Source: CAD feature listing. Evaluate the final solid. Frame: model axes, mm. A direction names the side the tool comes from. Round coordinates to 2 decimals unless told otherwise and drop trailing zeros. Loops run counter-clockwise (first coordinate to the right, second up) from the corner with the lowest first, then second, coordinate; pieces in that order, holes last. Notation, with made-up numbers: (77, 70.5) -> (125, 70.5) arc R9 cw to (125, 87.5) -> close; hole circle Ø8 at (45, 69). An arc over 180 degrees is marked (long way). Write item = value, one per line.
Autodesk Inventor part; units mm, degrees
ref_plane "YZ Plane" through (0, 0, 0) normal (1, 0, 0) x (0, 1, 0)
ref_plane "XZ Plane" through (0, 0, 0) normal (0, 1, 0) x (-1, 0, 0)
ref_plane "XY Plane" through (0, 0, 0) normal (0, 0, 1) x (1, 0, 0)
sketch "Sketch1" plane through (0, 0, 0) normal (0, 1, 0) x (-1, 0, 0)
  line L0 (0, 0) -> (31, 0)
  line L1 (31, 0) -> (31, -30)
  line L2 (31, -30) -> (28, -30)
  line L3 (28, -30) -> (28, -3)
  line L4 (28, -3) -> (0, -3)
  line L5 (0, -3) -> (0, 0) construction
  line L6 (0, 0) -> (-31, 0)
  line L7 (-31, 0) -> (-31, -30)
  line L8 (-31, -30) -> (-28, -30)
  line L9 (-28, -30) -> (-28, -3)
  line L10 (-28, -3) -> (0, -3)
  dimension "d0" = 31
  dimension "d1" = 30
  dimension "d2" = 3
  dimension "d3" = 27
extrude "Extrusion1" add sketch "Sketch1" along normal blind 20
sketch "Sketch2" plane through (31, 0, 0) normal (1, 0, 0) x (0, 0, -1)
  line L0 (30, 0) -> (0, 0) construction
  line L1 (0, 0) -> (15, 0) construction
  line L2 (15, 0) -> (15, 10) construction
  circle A0 centre (15, 10) radius 2.5
  dimension "d6" = 15
  dimension "d7" = 10
  dimension "d8" = 5
extrude "Extrusion2" cut sketch "Sketch2" against normal blind 70
fillet "Fillet1" radius 5 4 edges at (29.5, 20, -30) (29.5, 0, -30) (-29.5, 0, -30) (-29.5, 20, -30)
sketch "Sketch3" plane through (28, 0, -3) normal (0, 0, -1) x (-1, 0, 0)
  line L0 (28, 0) -> (28, 10) construction
  line L1 (28, 10) -> (48, 10) construction
  circle A0 centre (48, 10) radius 2
  circle A1 centre (8, 10) radius 2
  dimension "d12" = 10
  dimension "d13" = 20
  dimension "d14" = 4
extrude "Extrusion3" cut sketch "Sketch3" against normal blind 10
properties part number "Aligner"
1. Section query D-D (z = -15). Return the cut outline in (x, y).
Evaluation:
outline = (-31, 0) -> (-28, 0) -> (-28, 7.5) -> (-31, 7.5) -> close; (-31, 12.5) -> (-28, 12.5) -> (-28, 20) -> (-31, 20) -> close; (28, 0) -> (31, 0) -> (31, 7.5) -> (28, 7.5) -> close; (28, 12.5) -> (31, 12.5) -> (31, 20) -> (28, 20) -> close
2. Contact query for a flat-ended pin moving along its axis: pin 1 Ø4.5 at (x, y) = (-20, 10) entering from -Z. Output: stop coordinate, or through.
Evaluation:
pin_1 = -3
3. Line query: probe 1 along X at (y, z) = (9, -4.5); probe 2 along Y at (x, z) = (20, -1.7); probe 3 along Z at (x, y) = (10, 8). Output: solid intervals per line, ascending. Write a range as from..to.
Evaluation:
probe_1 = -31..-28, 28..31
probe_2 = 0..8, 12..20
probe_3 = -3..0
4. Section query A-A (z = -22.5). Return the cut outline in (x, y).
Evaluation:
outline = (-31, 0) -> (-28, 0) -> (-28, 20) -> (-31, 20) -> close; (28, 0) -> (31, 0) -> (31, 20) -> (28, 20) -> close
5. Section query B-B (x = -20). Return the cut outline in (y, z).
Evaluation:
outline = (0, -3) -> (8, -3) -> (8, 0) -> (0, 0) -> close; (12, -3) -> (20, -3) -> (20, 0) -> (12, 0) -> close
6. Mould query, pull axis X, two halves, no side actions, for faces 1 (the face through (-18.526, 11.352, -1.521)), 2 (the face through (-31, 10, -11)), 3 (the face through (31, 10, -11)), 4 (the face through (0, 0, -2)). Classes: released by +X, released by -X, zero draft, split by the parting line, or undercut.
Evaluation:
face_1 = undercut
face_2 = released by -X
face_3 = released by +X
face_4 = zero draft
7. Set-up query: faces 5 (the face through (0, 20, -2)), 6 (the face through (28, 8, -17)). Return all of +Z, -Z, +X, -X, +Y, -Y with unobstructed straight access to the full face (end or side cutting, diameter ignored); none if empty.
Evaluation:
face_5 = +Z, -Z, +X, -X, +Y
face_6 = -Z, +Y, -Y
8. Section query C-C (y = 10). Return the cut outline in (x, z).
Evaluation:
outline = (-31, -30) -> (-28, -30) -> (-28, -17.5) -> (-31, -17.5) -> close; (-31, -12.5) -> (-28, -12.5) -> (-28, -3) -> (-22, -3) -> (-22, 0) -> (-31, 0) -> close; (-18, -3) -> (18, -3) -> (18, 0) -> (-18, 0) -> close; (22, -3) -> (28, -3) -> (28, -12.5) -> (31, -12.5) -> (31, 0) -> (22, 0) -> close; (28, -30) -> (31, -30) -> (31, -17.5) -> (28, -17.5) -> close
